The drawing under review shows one solid part. Ordinate dimensions are in mm from its lowest x, y, z. A direction names the side the tool comes from. Give positions to 0.01 mm unless a question says otherwise; leave off trailing zeros. Order: outer loops, then holes, each group sorted by start corner. A loop starts at its lowest first (then second) coordinate and runs counter-clockwise, first axis right, second up. Notation, with made-up numbers: (39.5, -32) - (50.5, -32) arc R17 cw to (50.5, -21) - close; hole circle Ø7 at (46, 75). An arc over 180 degrees is marked (long way). Use CSV: the item, a comma, the result in double quotes. Start each with the question number.
1. Take a section at A-A, the plane x = 125. State the section outline as (y, z) points, then the cut area to 3 significant figures.
2. To check wall thickness, follow line 1 (X direction, y = 33.5, z = 8.5); line 2 (X direction, y = 44, z = 26); line 3 (X direction, y = 56, z = 18.5). State the ranges of each line that lie inside material, in increasing order. Write a range as [from, to].
3. Take a section at B-B, the plane z = 41.5. State the section outline as (x, y) points, then the cut area to 3 significant figures.
4. For pin 1 (2 mm diameter, centred on x = 202.5, y = 44, fed in from +Z); pin 2 (15.5 mm diameter, centred on x = 125, z = 24.85, fed in from -Y), all flat-tipped, find the tip position at first contact; note any pin that passes through.
5. Machinability: for the marked faces 5 and 6, which of the approach directions +Z, -Z, +X, -X, +Y, -Y give a long, thin tool a straight path to every point of the face, cutting with its end or side? Answer none if there is none.
6. Take a section at C-C, the plane x = 46. State the section outline as (y, z) points.
7. Draft analysis for pull direction Y (two halves, no side actions). For the marked faces 1, 2, 3 and 4, state which applies: released by +Y, released by -Y, zero draft, split by the parting line, or undercut.
8. Take a section at D-D, the plane y = 53. State the section outline as (x, z) points.
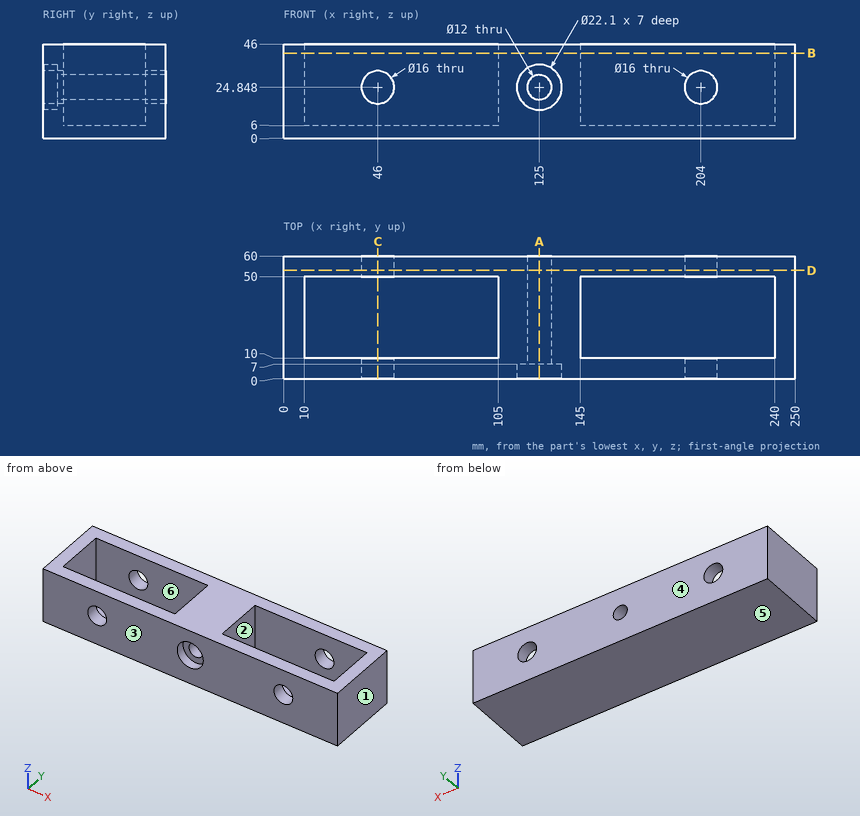
Determined:
1,outline,"(0, 0) - (60, 0) - (60, 18.85) - (7, 18.85) - (7, 13.8) - (0, 13.8) - close; (0, 35.9) - (7, 35.9) - (7, 30.85) - (60, 30.85) - (60, 46) - (0, 46) - close"
1,area,"1,970 mm²"
2,line 1,"x = [0, 10], [105, 145], [240, 250]"
2,line 2,"x = [0, 10], [105, 119.11], [130.89, 145], [240, 250]"
2,line 3,"x = [0, 41.13], [50.87, 199.13], [208.87, 250]"
3,outline,"(0, 0) - (250, 0) - (250, 60) - (0, 60) - close; hole (10, 10) - (105, 10) - (105, 50) - (10, 50) - close; hole (145, 10) - (240, 10) - (240, 50) - (145, 50) - close"
3,area,"7,400 mm²"
4,pin 1,"stops at z = 6"
4,pin 2,"stops at y = 7"
5,face 5,"-Z, +X, -X, +Y, -Y"
5,face 6,"+Z"
6,outline,"(0, 0) - (60, 0) - (60, 16.85) - (50, 16.85) - (50, 6) - (10, 6) - (10, 16.85) - (0, 16.85) - close; (0, 32.85) - (10, 32.85) - (10, 46) - (0, 46) - close; (50, 32.85) - (60, 32.85) - (60, 46) - (50, 46) - close"
7,face 1,"zero draft"
7,face 2,"undercut"
7,face 3,"released by -Y"
7,face 4,"released by +Y"
8,outline,"(0, 0) - (250, 0) - (250, 46) - (0, 46) - close; hole circle Ø16 at (46, 24.85); hole circle Ø12 at (125, 24.85); hole circle Ø16 at (204, 24.85)"
